Verification items for this drawing (mm, ordinates from the low corner). A direction names the side the tool comes from. Round coordinates to 2 decimals unless told otherwise and drop trailing zeros. Loops run counter-clockwise (first coordinate to the right, second up) from the corner with the lowest first, then second, coordinate; pieces in that order, holes last. Notation, with made-up numbers: M 71,-39.5 L 129,-39.5 A29 cw 129,-5.5 Z; hole C -28,1.5 d11. An arc over 180 degrees is marked long. Write item = value, one per line. Start each with the question number.
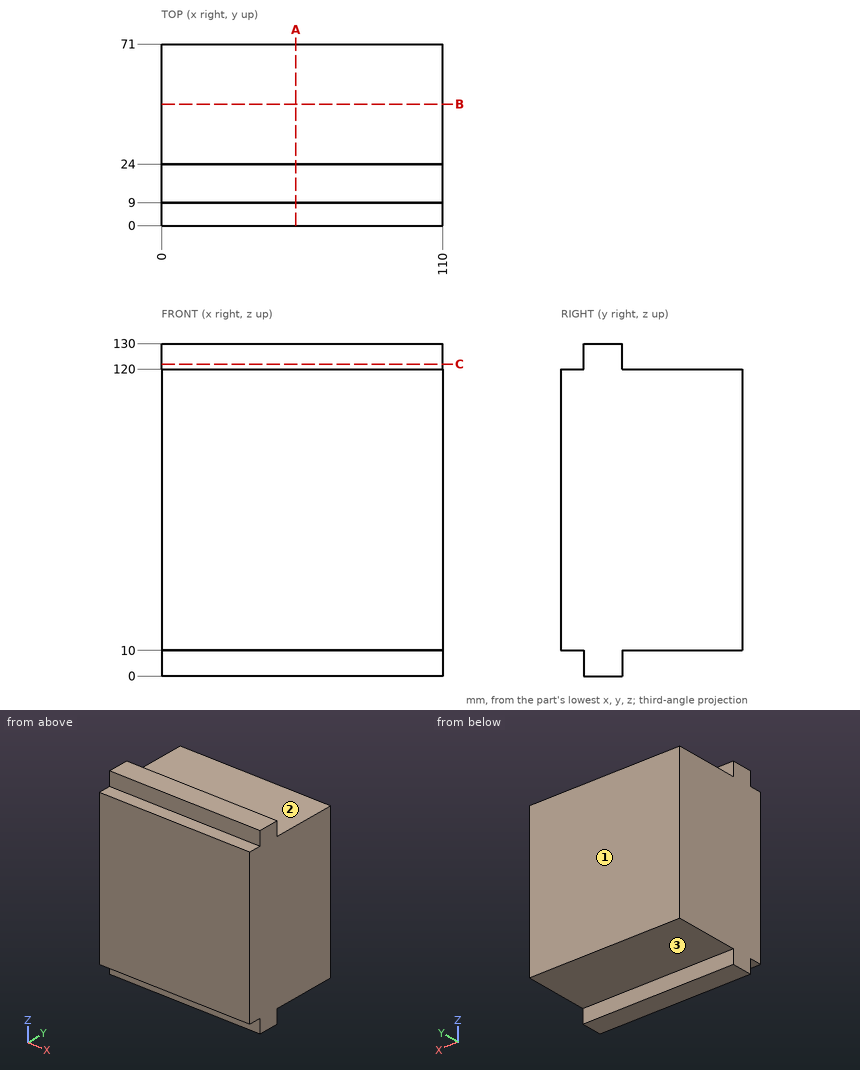
1. Section check B-B, the plane y = 47.5. Enter the section's corners in (x, z).
2. Gauge pin test, flat ends, axial feed: P1, Ø3, axis at x = 50.5, z = 126, coming from the +Y side; P2, Ø2.5, axis at x = 57.5, y = 6, coming from the -Z side; P3, Ø8, axis at x = 61.5, z = 125, coming from the -Y side. Record the tip position at first contact, or that the pin passes through.
3. Section check A-A, the plane x = 52.5. Enter the section's corners in (y, z), and give its area (3 significant figures).
4. Section check C-C, the plane z = 122. Enter the section's corners in (x, y), and give its area (3 significant figures).
5. Thickness scan on line 1 (Z direction, x = 28, y = 63.5); line 2 (Y direction, x = 77, z = 6). Record the ranges inside material, lowest first.
6. Tool access check on the marked faces 1, 2 and 3. Record the directions out of +Z, -Z, +X, -X, +Y, -Y that give a thin tool (end or side, any length) a straight path to the whole face; none if there is none.
Computed values:
q1.outline = M 0,10 L 110,10 L 110,120 L 0,120 Z
q2.P1 = 24
q2.P2 = 10
q2.P3 = 9
q3.outline = M 0,10 L 9,10 L 9,0 L 24,0 L 24,10 L 71,10 L 71,120 L 24,120 L 24,130 L 9,130 L 9,120 L 0,120 Z
q3.area = 8,110 mm2
q4.outline = M 0,9 L 110,9 L 110,24 L 0,24 Z
q4.area = 1,650 mm2
q5.line_1 = 10 to 120
q5.line_2 = 9 to 24
q6.face_1 = +Z, -Z, +X, -X, +Y
q6.face_2 = +Z, +X, -X, +Y
q6.face_3 = -Z, +X, -X, +Y
